Geometry: see drawing. Coordinates: mm, zero at the bounding-box minimum. A direction names the side the tool comes from. Give positions to 0.01 mm unless a question says otherwise; leave off trailing zeros. Write each loop counter-clockwise with the first axis right and the second up, starting at its lowest first coordinate (ties: lowest second). Pieces come first, ordered by that corner, then holes. Notation, with made-up numbers: M 70.5,51 L 82.5,51 A23 cw 82.5,73 Z; hole C 60,-32 d1. An arc over 180 degrees is marked long. Use a Markdown table: item, result. Add a question column.
(1) Draft query along Y for the marked faces 1 and 2. Return one class per face: released by +Y, released by -Y, zero draft, split by the parting line, or undercut.
(2) Pin query (flat end, axial travel): pin 1 Ø2 at (y, z) = (2.5, 7) entering from +X; pin 2 Ø1 at (y, z) = (14.5, 2.5) entering from +X; pin 3 Ø2 at (x, y) = (2, 23) entering from -Z. Return the tip coordinate at first contact, or that it passes through.
(3) Cut plane D-D (z = 5). Output: boundary loops of the cut face in (x, y), plus the area to 3 significant figures.
(4) Cut plane B-B (y = 22.5). Output: boundary loops of the cut face in (x, z).
(5) Cut plane C-C (x = 2.5). Output: boundary loops of the cut face in (y, z).
(6) Material intervals for L1, parallel to Y at x = 2.45, z = 3; L2, parallel to Y at x = 2.65, z = 1; L3, parallel to Z at x = 0.25, y = 23.5, sorted ascending.
(7) Reachability of the marked faces 3, 4 and 5 from +Z, -Z, +X, -X, +Y, -Y: full face, straight path, thin tool, end or side. Return the list, or none.
(8) Cut plane A-A (z = 1.25). Output: boundary loops of the cut face in (x, y).
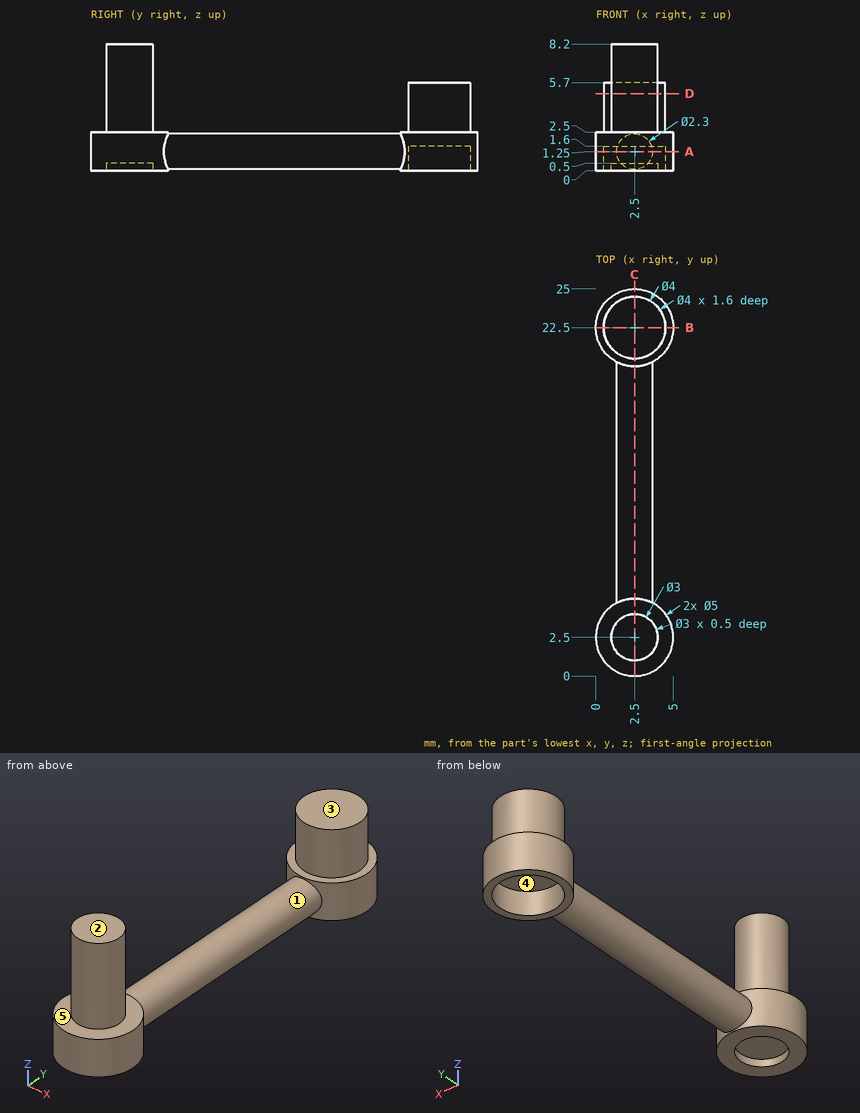
Answer list:
| question | item | result |
|---|---|---|
| 1 | face 1 | undercut |
| 1 | face 2 | zero draft |
| 2 | pin 1 | x = 4 |
| 2 | pin 2 | x = 3.37 |
| 2 | pin 3 | z = 1.6 |
| 3 | outline | C 2.5,22.5 d4; C 2.5,2.5 d3 |
| 3 | area | 19.6 mm² |
| 4 | outline | M 0,0 L 0.5,0 L 0.5,1.6 L 4.5,1.6 L 4.5,0 L 5,0 L 5,2.5 L 4.5,2.5 L 4.5,5.7 L 0.5,5.7 L 0.5,2.5 L 0,2.5 Z |
| 5 | outline | M 0,0 L 1,0 L 1,0.5 L 4,0.5 L 4,0 L 5,0 L 5,0.1 L 20,0.1 L 20,0 L 20.5,0 L 20.5,1.6 L 24.5,1.6 L 24.5,0 L 25,0 L 25,2.5 L 24.5,2.5 L 24.5,5.7 L 20.5,5.7 L 20.5,2.5 L 20,2.5 L 20,2.4 L 5,2.4 L 5,2.5 L 4,2.5 L 4,8.2 L 1,8.2 L 1,2.5 L 0,2.5 Z |
| 6 | L1 | 1 to 4, 20.5 to 24.5 |
| 6 | L2 | 0 to 20.51, 24.49 to 25 |
| 6 | L3 | 0 to 2.5 |
| 7 | face 3 | +Z, +X, -X, +Y |
| 7 | face 4 | -Z |
| 7 | face 5 | +Z |
| 8 | outline | M 1.35,4.72 A2.5 ccw long 3.65,4.72 L 3.65,20.28 A2.5 ccw long 1.35,20.28 Z; hole C 2.5,22.5 d4 |
